Design review of the part built by this model. Coordinates are the model's own, in mm. Face numbers are marked on the shaded views. Round coordinates to 2 decimals unless told otherwise and drop trailing zeros. Loops run counter-clockwise (first coordinate to the right, second up) from the corner with the lowest first, then second, coordinate; pieces in that order, holes last. Notation, with made-up numbers: M 13,76.5 L 26,76.5 A27 cw 26,97.5 Z; hole C 68.25,74 d1. An arc over 180 degrees is marked long. Use a Markdown table: item, result.
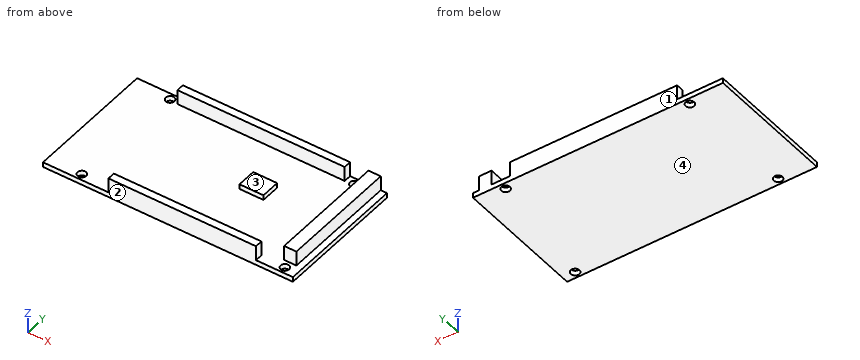
from build123d import *

# Parameters (mm, degrees)
SKETCH_1_W      = 101.6
SKETCH_1_H      = 53.34
SKETCH_1_R      = 1.75
EXTRUDE_1_DEPTH = 2
SKETCH_2_W      = 68
SKETCH_2_H      = 3.07
SKETCH_2_W_2    = 60
SKETCH_2_W_3    = 5
SKETCH_2_H_2    = 47.81
EXTRUDE_2_DEPTH = 6
SKETCH_3_W      = 9.737104959
SKETCH_3_H      = 7.755742322
EXTRUDE_3_DEPTH = 2


with BuildPart() as part:
    # 草图1 → 凸台-拉伸1 (new body)
    with BuildSketch(Plane.XY):
        Rectangle(SKETCH_1_W, SKETCH_1_H)
        with Locations((-35.56, 24.13)):
            Circle(SKETCH_1_R, mode=Mode.SUBTRACT)
        with Locations((-36.83, -24.13)):
            Circle(SKETCH_1_R, mode=Mode.SUBTRACT)
        with Locations((45.72, -24.13)):
            Circle(SKETCH_1_R, mode=Mode.SUBTRACT)
        with Locations((39.37, 24.13)):
            Circle(SKETCH_1_R, mode=Mode.SUBTRACT)
    extrude(amount=EXTRUDE_1_DEPTH)

    # 草图2 → 凸台-拉伸2 (add)
    with BuildSketch(Plane.XY.offset(2)):
        with Locations((1.8, 25.135)):
            Rectangle(SKETCH_2_W, SKETCH_2_H)
        with Locations((5.8, -25.135)):
            Rectangle(SKETCH_2_W_2, SKETCH_2_H)
        with Locations((45.76, 2.765)):
            Rectangle(SKETCH_2_W_3, SKETCH_2_H_2)
    extrude(amount=EXTRUDE_2_DEPTH)

    # 草图3 → 凸台-拉伸3 (add)
    with BuildSketch(Plane.XY.offset(2)):
        with Locations((14.832089241, 3.877871161)):
            Rectangle(SKETCH_3_W, SKETCH_3_H)
    extrude(amount=EXTRUDE_3_DEPTH)


solid = part.part
1. Take a section at A-A on x = 45.72. Give the boundary of the cut face in (y, z).
Check values:
| item | result |
|---|---|
| outline | M -26.67,0 L -25.88,0 L -25.88,2 L -26.67,2 Z; M -22.38,0 L 26.67,0 L 26.67,8 L -21.14,8 L -21.14,2 L -22.38,2 Z |
2. Take a section at C-C on x = -16. Give the boundary of the cut face in (y, z).
Check values:
| item | result |
|---|---|
| outline | M -26.67,0 L 26.67,0 L 26.67,8 L 23.6,8 L 23.6,2 L -23.6,2 L -23.6,8 L -26.67,8 Z |
3. Take a section at B-B on z = 6. Give the boundary of the cut face in (x, y), and give its area (3 significant figures).
Check values:
| item | result |
|---|---|
| outline | M -32.2,23.6 L 35.8,23.6 L 35.8,26.67 L -32.2,26.67 Z; M -24.2,-26.67 L 35.8,-26.67 L 35.8,-23.6 L -24.2,-23.6 Z; M 43.26,-21.14 L 48.26,-21.14 L 48.26,26.67 L 43.26,26.67 Z |
| area | 632 mm² |
4. Take a section at D-D on y = -10. Give the boundary of the cut face in (x, z).
Check values:
| item | result |
|---|---|
| outline | M -50.8,0 L 50.8,0 L 50.8,2 L 48.26,2 L 48.26,8 L 43.26,8 L 43.26,2 L -50.8,2 Z |
5. The part is to be moulded in two halves that separate along Y. For the marked faces 1, 2, 3 and 4, say which applies: pulls with the +Y half, pulls with the -Y half, needs draft (parallel to the pull), parting line crosses it, or undercut.
Check values:
| item | result |
|---|---|
| face 1 | pulls with the +Y half |
| face 2 | pulls with the -Y half |
| face 3 | undercut |
| face 4 | needs draft |
6. Wall thickness on line 1 along Y through (x, z) = (11, 3.25); line 2 along Y through (x, z) = (45.72, 1.45); line 3 along Y through (x, z) = (-36.83, 0.6): over which ranges is each line inside the solid? List them lowest first. Write a range as from..to.
Check values:
| item | result |
|---|---|
| line 1 | y = -26.67..-23.6, 0..7.76, 23.6..26.67 |
| line 2 | y = -26.67..-25.88, -22.38..26.67 |
| line 3 | y = -26.67..-25.88, -22.38..22.93, 25.33..26.67 |
7. Insertion check: pin 1 (2.5 mm diameter, centred on y = -25.5, z = 6.5, fed in from -X); pin 2 (3 mm diameter, centred on y = -7.5, z = 5.5, fed in from -X); pin 3 (2.5 mm diameter, centred on y = 25, z = 4, fed in from -X). Each pin has a flat end and moves straight along its axis. Give the tip position at first contact, or say it passes through.
Check values:
| item | result |
|---|---|
| pin 1 | stops at x = -24.2 |
| pin 2 | stops at x = 43.26 |
| pin 3 | stops at x = -32.2 |
